```python
from build123d import *

# Parameters (mm, degrees)
F0_W     = 50.8
F0_H     = 19.05
F1_DEPTH = 1123.95
F2_W     = 122.435573
F2_H     = 50.8
F2_W_2   = 93.867282
F2_W_3   = 145.562325
F2_W_4   = 343.160421
F2_H_2   = 127
F3_DEPTH = 25.4
F4_R     = 0.79375
F5_DEPTH = 25.4
F6_R     = 4.7625
F7_DEPTH = 25.4


with BuildPart() as f1:
    # F0 (on Top) → F1 (new body)
    with BuildSketch(Plane.XY):
        Rectangle(F0_W, F0_H)
    extrude(amount=F1_DEPTH)

    # F2 (on Front) → F3 (cut)
    with BuildSketch(Plane.XZ):
        with Locations((22.446524, 25.4)):
            Rectangle(F2_W, F2_H)
        with Locations((2.720783, 755.65)):
            Rectangle(F2_W_2, F2_H)
        with Locations((-1.360391, 482.6)):
            Rectangle(F2_W_3, F2_H)
        with Locations((-38.781822, 1060.45)):
            Rectangle(F2_W_4, F2_H_2)
    extrude(amount=F3_DEPTH, mode=Mode.SUBTRACT)

    # F4 (on Front) → F5 (cut)
    with BuildSketch(Plane.XZ):
        with Locations((9.525, 101.6)):
            Circle(F4_R)
        with Locations((9.525, 155.575)):
            Circle(F4_R)
        with Locations((9.525, 625.475)):
            Circle(F4_R)
        with Locations((9.525, 679.45)):
            Circle(F4_R)
        with Locations((-9.525, 625.475)):
            Circle(F4_R)
        with Locations((-9.525, 679.45)):
            Circle(F4_R)
        with Locations((-9.525, 101.6)):
            Circle(F4_R)
        with Locations((-9.525, 155.575)):
            Circle(F4_R)
    extrude(amount=-F5_DEPTH, mode=Mode.SUBTRACT)

    # F6 (on Front) → F7 (cut)
    with BuildSketch(Plane.XZ):
        with Locations((15.875, 76.2)):
            Circle(F6_R)
        with Locations((-15.875, 76.2)):
            Circle(F6_R)
        with Locations((-15.875, 304.8)):
            Circle(F6_R)
    extrude(amount=F7_DEPTH, mode=Mode.SUBTRACT)


solid = f1.part
```
Geometry check sheet. Reference: the model listing, model coordinates, mm. A direction names the side the tool comes from. Give positions to 0.01 mm unless a question says otherwise; leave off trailing zeros. Loops run counter-clockwise (first coordinate to the right, second up) from the corner with the lowest first, then second, coordinate; pieces in that order, holes last. Notation, with made-up numbers: M 15,28 L 37,28 A29 cw 37,66 Z; hole C 0,-6.75 d5. An arc over 180 degrees is marked long. Answer as CSV lines item,"result".
Item 1: Cross-section at C-C on z = 1044. Record the cut outline in (x, y) (3 decimals).
Values:
outline,"M -25.4,0 L 25.4,0 L 25.4,9.525 L -25.4,9.525 Z"
Item 2: Access from +Z, -Z, +X, -X, +Y, -Y to the whole of each face (thin tool, end or side, straight path). Record for faces 1 (the flat face through (0, 0, 1061)), 2 (the flat face through (0, 9.525, 554)), 3 (the flat face through (0, 0, 26)), 4 (the flat face through (-25.4, 0, 554)), 5 (the flat face through (0, 0, 756)).
Values:
face 1,"+Z, +X, -X, -Y"
face 2,"+Z, -Z, +X, -X, +Y"
face 3,"-Z, +X, -X, -Y"
face 4,"+Z, -Z, -X, +Y, -Y"
face 5,"+X, -X, -Y"
Item 3: Cross-section at A-A on y = -5. Count the separate pieces of the cut face and the enclosed holes in it, and give its area (3 significant figures).
Values:
separate pieces,"3"
enclosed holes,"3"
area,"42,700 mm²"
Item 4: Cross-section at B-B on x = -0.5. Record the cut outline in (y, z) (3 decimals).
Values:
outline,"M -9.525,50.8 L 0,50.8 L 0,0 L 9.525,0 L 9.525,1123.95 L 0,1123.95 L 0,996.95 L -9.525,996.95 L -9.525,781.05 L 0,781.05 L 0,730.25 L -9.525,730.25 L -9.525,508 L 0,508 L 0,457.2 L -9.525,457.2 Z"
Item 5: Material ranges on line 1 (Z direction, x = -22, y = -5); line 2 (X direction, y = 3, z = 101.6); line 3 (Z direction, x = -10, y = 6), recorded low to high.
Values:
line 1,"z = 50.8 to 457.2, 508 to 730.25, 781.05 to 996.95"
line 2,"x = -25.4 to -10.32, -8.73 to 8.73, 10.32 to 25.4"
line 3,"z = 0 to 100.96, 102.24 to 154.94, 156.21 to 624.84, 626.11 to 678.81, 680.09 to 1123.95"
Item 6: Depth check by flat-ended pin: P1, Ø5.5, axis at x = 15.875, z = 76.2, coming from the -Y side; P2, Ø1.4, axis at x = 9.525, z = 625.475, coming from the +Y side; P3, Ø5, axis at x = -10, y = -3, coming from the +Z side. Enter the tip coordinate at first touch or a pass-through.
Values:
P1,"stops at y = 0"
P2,"stops at y = 0"
P3,"stops at z = 996.95"
Item 7: Release check for a two-part mould opening along Z. For faces 6 (the flat face through (0, 0, 483)), 7 (the flat face through (0, -9.525, 887)) record: pulls with the +Z half, pulls with the -Z half, needs draft (parallel to the pull), parting line crosses it, or undercut.
Values:
face 6,"undercut"
face 7,"needs draft"
